Could you check a few things on this drawing? It's one solid part, dimensions in mm from its lowest x, y, z. Give positions to 0.01 mm unless a question says otherwise; leave off trailing zeros. Order: outer loops, then holes, each group sorted by start corner. A loop starts at its lowest first (then second) coordinate and runs counter-clockwise, first axis right, second up. Notation, with made-up numbers: M -27.5,40 L -14.5,40 A26 cw -14.5,69 Z; hole C 15,-11.5 d5. An arc over 180 degrees is marked long. One line per item, written item: value. Start each with the question number.
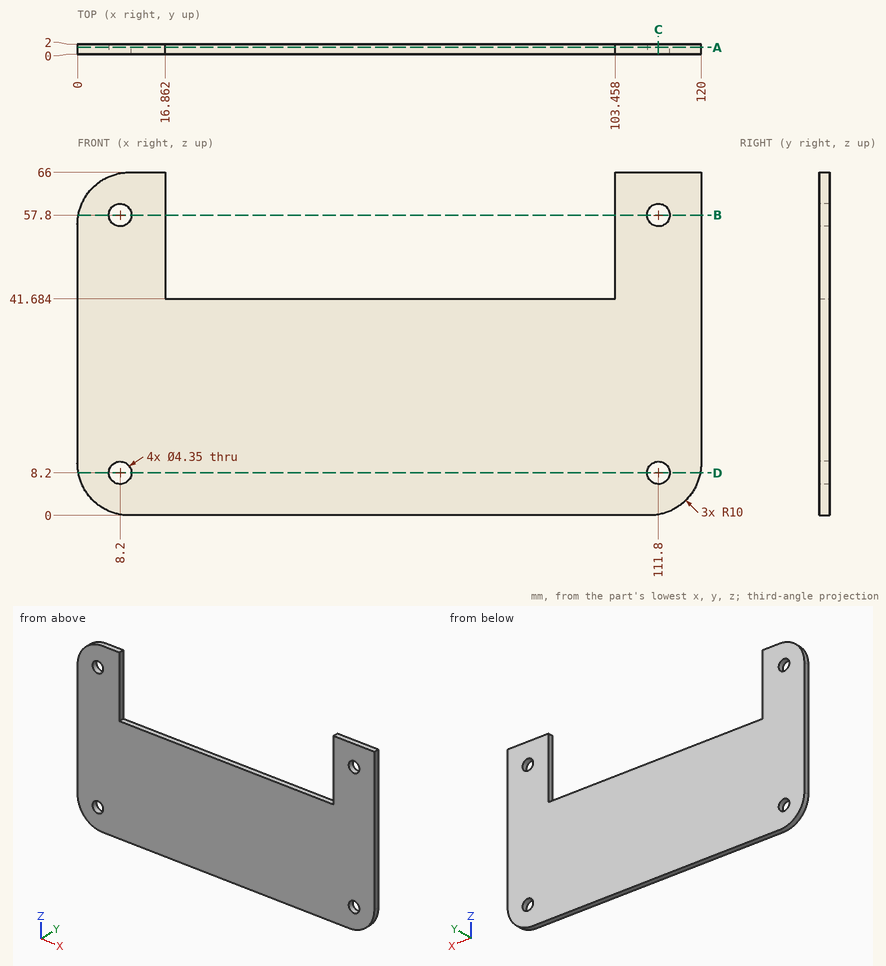
Item 1: Please list where these lines run through material, in increasing order: probe 1 along X at (y, z) = (1.3, 57.8) (1 decimal); probe 2 along X at (y, z) = (0.6, 47); probe 3 along X at (y, z) = (0.85, 10). Write a range as [from, to].
Item 2: I want a section at C-C on x = 111.8. Write out the boundary of the cut face in (y, z) (1 decimal).
Item 3: I want a section at A-A on y = 1.35. Count the separate pieces of the cut face and the enclosed holes in it, plus the area to 3 significant figures.
Item 4: Will this pin go through, and if not, where does the flat tip stop? P1, Ø1, axis at x = 64, y = 1, coming from the +Z side.
Item 5: I want a section at B-B on z = 57.8. Write out the boundary of the cut face in (x, y) (1 decimal).
Item 6: I want a section at D-D on z = 8.2. Write out the boundary of the cut face in (x, y) (1 decimal).
Answer below:
1. probe 1: x = [0.2, 6], [10.4, 16.9], [103.5, 109.6], [114, 120]
1. probe 2: x = [0, 16.86], [103.46, 120]
1. probe 3: x = [0, 6.98], [9.42, 110.58], [113.02, 120]
2. outline: M 0,0.2 L 2,0.2 L 2,6 L 0,6 Z; M 0,10.4 L 2,10.4 L 2,55.6 L 0,55.6 Z; M 0,60 L 2,60 L 2,66 L 0,66 Z
3. separate pieces: 1
3. enclosed holes: 4
3. area: 5,690 mm²
4. P1: stops at z = 41.68
5. outline: M 0.2,0 L 6,0 L 6,2 L 0.2,2 Z; M 10.4,0 L 16.9,0 L 16.9,2 L 10.4,2 Z; M 103.5,0 L 109.6,0 L 109.6,2 L 103.5,2 Z; M 114,0 L 120,0 L 120,2 L 114,2 Z
6. outline: M 0.2,0 L 6,0 L 6,2 L 0.2,2 Z; M 10.4,0 L 109.6,0 L 109.6,2 L 10.4,2 Z; M 114,0 L 119.8,0 L 119.8,2 L 114,2 Z
